Build history of the part. All positions in model axes, mm. A direction names the side the tool comes from. Give positions to 0.01 mm unless a question says otherwise; leave off trailing zeros. Write each loop counter-clockwise with the first axis right and the second up, starting at its lowest first coordinate (ties: lowest second). Pieces come first, ordered by that corner, then holes. Notation, with made-up numbers: M 12.25,2.5 L 62.25,2.5 A20 cw 62.25,35.5 Z; hole C -36,-32 d2. An arc over 180 degrees is marked long. Return JSON: item names as keys, results as strings. Group by question number.
Q1. Band-saw the part on C-C, the plane y = -51.5. Give the cut face in (x, z).
Q2. Pull direction X, two halves, no side cores. Call faces 1 (the flat face through (0, -61.7, -6.5)), 2 (the cylindrical face through (0.315, -61, -16.764)), 3 (the flat face through (-22.5, -57, -19)), 4 (the flat face through (4, -44, -19)): +X half, -X half, draft (parallel to the pull), parting line (faces both ways), or undercut.
Q3. Band-saw the part on B-B, the plane x = -6.5. Give the cut face in (y, z).
Q4. Band-saw the part on D-D, the plane z = -12.5. Give the cut face in (x, y).
Q5. Band-saw the part on A-A, the plane z = -4. Give the cut face in (x, y) (3 decimals), then the cut area to 3 significant figures.
Q6. Tool access for faces 5 (the cylindrical face through (13.9, -62.01, -4.91)), 6 (the flat face through (-14, -63, -4.5)), 7 (the flat face through (0, -45.893, -19)), 8 (the flat face through (14, -63, -4.5)): list every direction of +Z, -Z, +X, -X, +Y, -Y with a clear straight run to the whole face (end or side of a thin tool).
Q7. Flat gauge pins, fed straight in: pin 1 Ø1.9 at (y, z) = (-61, -3.5) entering from -X; pin 2 Ø1.7 at (x, z) = (-2.5, -3.5) entering from +Y; pin 3 Ø1.8 at (x, y) = (-13, -62.5) entering from +Z; pin 4 Ø2.5 at (x, z) = (0, -4) entering from -Y. Where does each tip first touch, or does it go through?
Q8. Wall check: probe 1 along Z at (x, y) = (0, -61.2) (3 decimals); probe 2 along Z at (x, y) = (0, -60.4) (3 decimals); probe 3 along X at (y, z) = (-63.05, -4). Give the ranges that are in metal, low to high.
from build123d import *

# Parameters (mm, degrees)
MODEL_R                   = 8.35
RESSALTO_EXTRUS_O2_DEPTH  = 4
ESBO_O5_W                 = 2
ESBO_O5_H                 = 24
RESSALTO_EXTRUS_O3_DEPTH  = 20
ESBO_O6_OUTSIDE_W         = 30.002
ESBO_O6_OUTSIDE_H         = 34.002
ESBO_O6_OUTSIDE_R         = 13
CORTE_EXTRUS_O1_DEPTH     = 72.292987034
CORTE_EXTRUS_O2_DEPTH     = 72.292987124
RESSALTO_EXTRUS_O4_DEPTH  = 4
CORTE_EXTRUS_O3_DEPTH     = 38.486664414
RESSALTO_EXTRUS_O5_START  = 0.5
RESSALTO_EXTRUS_O5_DEPTH  = 45
RESSALTO_EXTRUS_O6_START  = 0.5
ESBO_O14_R                = 2.115
RESSALTO_EXTRUS_O6_DEPTH  = 3.779219
CORTE_EXTRUS_O4_DEPTH     = 10.1
CORTE_EXTRUS_O7_DEPTH     = 10
ESBO_O17_R                = 3.5
CORTE_EXTRUS_O8_DEPTH     = 2
CORTE_EXTRUS_O11_REACH    = 75.217
ESBO_O19_W                = 67.006666236
ESBO_O19_H                = 28.204946311
CORTE_EXTRUS_O9_DEPTH     = 52.948283002
CORPO_MOVER_COPIAR2_ANGLE = 180


with BuildPart() as part:
    # Model → Ressalto-extrusão2 (new body)
    with BuildSketch(Plane.XY):
        Polygon((0, 44.200000002), (0, 59.200000002), (-5.55, 59.200000002), (-5.55, 63.700000002), (-23, 63.700000002), (-23, 39.700000002), (-5.55, 39.700000002), (-5.55, 44.200000002), align=None)
        with Locations((-13.5, 51.700000002)):
            Circle(MODEL_R, mode=Mode.SUBTRACT)
    extrude(amount=RESSALTO_EXTRUS_O2_DEPTH)

    # Esboço5 → Ressalto-extrusão3 (add)
    with BuildSketch(Plane(origin=(0, 0, 0), x_dir=(-1, 0, 0), z_dir=(0, 0, -1))):
        with Locations((24, 51.700000002)):
            Rectangle(ESBO_O5_W, ESBO_O5_H)
    extrude(amount=-RESSALTO_EXTRUS_O3_DEPTH)

    # Esboço6 outside → Corte-extrusão1 (cut, through all)
    with BuildSketch(Plane.ZY.offset(25)):
        with Locations((10, 51.7)):
            Rectangle(ESBO_O6_OUTSIDE_W, ESBO_O6_OUTSIDE_H)
        with Locations((10, 51.700000002)):
            Circle(ESBO_O6_OUTSIDE_R, mode=Mode.SUBTRACT)
    extrude(amount=-CORTE_EXTRUS_O1_DEPTH, mode=Mode.SUBTRACT)

    # Esboço8 → Corte-extrusão2 (cut, through all)
    with BuildSketch(Plane.ZY.offset(25)):
        Polygon((7.885, 51.700000002), (10, 49.585000002), (12.115, 51.700000002), (10, 53.815000002), align=None)
    extrude(amount=-CORTE_EXTRUS_O2_DEPTH, mode=Mode.SUBTRACT)

    # Espelhar1: part across plane


with BuildPart() as part_1:
    add(part.part)
    add(part.part.mirror(Plane(origin=(0, 44.200000002, 4), x_dir=(0, 0, 1), z_dir=(-1, 0, 0))))

    # Esboço9 → Ressalto-extrusão4 (add)
    with BuildSketch(Plane.XY.offset(4)):
        Polygon((0, 59.200000002), (4, 59.200000002), (4, 44.200000002), (-4, 44.200000002), (-4, 59.200000002), align=None)
    extrude(amount=RESSALTO_EXTRUS_O4_DEPTH)

    # Esboço10 → Corte-extrusão3 (cut, through all)
    with BuildSketch(Plane(origin=(0, 59.200000002, 0), x_dir=(1, 0, 0), z_dir=(0, 1, 0))):
        Polygon((0, -1.885), (-2.115, -4), (0, -6.115), (2.115, -4), align=None)
    extrude(amount=-CORTE_EXTRUS_O3_DEPTH, mode=Mode.SUBTRACT)


with BuildPart() as body_2:
    # Esboço13 → Ressalto-extrusão5 (new body)
    with BuildSketch(Plane.ZY.offset(-23).offset(RESSALTO_EXTRUS_O5_START)):
        with BuildLine():
            Line((18.5, 43.95403331), (18.5, 59.445966694))
            ThreePointArc((18.5, 59.445966694), (16.73742843, 61.019713418), (14.69041576, 62.200000002))
            Line((14.69041576, 62.200000002), (5.30958424, 62.200000002))
            ThreePointArc((5.30958424, 62.200000002), (4.900858659, 62.0077038), (4.5, 61.79950494))
            Line((4.5, 61.79950494), (4.5, 63.479218991))
            ThreePointArc((4.5, 63.479218991), (4.748839551, 63.592237552), (5, 63.700000002))
            Line((5, 63.700000002), (15, 63.700000002))
            ThreePointArc((15, 63.700000002), (17.724005232, 62.156564599), (20, 60.006623865))
            Line((20, 60.006623865), (20, 43.393376139))
            ThreePointArc((20, 43.393376139), (19.281560672, 42.597657914), (18.5, 41.863842216))
            Line((18.5, 41.863842216), (18.5, 43.95403331))
        make_face()
    extrude(amount=RESSALTO_EXTRUS_O5_DEPTH)

    # Esboço14 → Ressalto-extrusão6 (add)
    with BuildSketch(Plane(origin=(0, 59.200000002, 0), x_dir=(1, 0, 0), z_dir=(0, 1, 0)).offset(RESSALTO_EXTRUS_O6_START)):
        Polygon((5.05, -4), (5.05, -8), (5.05, -9.5), (-5.05, -9.5), (-5.05, -8), (-5.05, -4), (-5.05, -0.5), (5.05, -0.5), align=None)
        with Locations(Location((0, -4, 0), (0, 0, 346.325447319))):
            Circle(ESBO_O14_R, mode=Mode.SUBTRACT)
    extrude(amount=RESSALTO_EXTRUS_O6_DEPTH)

    # Esboço15 → Corte-extrusão4 (cut)
    with BuildSketch(Plane(origin=(5.05, 0, 0), x_dir=(0, 0, -1), z_dir=(1, 0, 0))):
        with BuildLine():
            Line((-5.561651151, 63.918881272), (-4.5, 63.918881272))
            Line((-4.5, 63.918881272), (-4.5, 64.979109715))
            Line((-4.5, 64.979109715), (0, 64.979109715))
            Line((0, 64.979109715), (0, 60.006623865))
            ThreePointArc((0, 60.006623865), (-2.520500092, 62.332830346), (-5.561651151, 63.918881272))
        make_face()
    extrude(amount=-CORTE_EXTRUS_O4_DEPTH, mode=Mode.SUBTRACT)

    # Esboço18 → Corte-extrusão7 (cut)
    with BuildSketch(Plane.XY.offset(20)):
        Polygon((-4, 45.893376139), (0, 45.893376139), (4, 45.893376139), (4, 37.813192245), (-4, 37.813192245), align=None)
    extrude(amount=-CORTE_EXTRUS_O7_DEPTH, mode=Mode.SUBTRACT)

    # Esboço17 → Corte-extrusão8 (cut)
    with BuildSketch(Plane(origin=(0, 63.700000002, 0), x_dir=(1, 0, 0), z_dir=(0, 1, 0))):
        with Locations((0, -4)):
            Circle(ESBO_O17_R)
    extrude(amount=-CORTE_EXTRUS_O8_DEPTH, mode=Mode.SUBTRACT)

    # Corte-extrusão11: up to this face of the body (flat: up to its plane)
    corte_extrus_o11_end = Plane(body_2.part.faces().sort_by_distance((-5.05, 61.009194207, 5.162360776))[0])
    # Esboço21 → Corte-extrusão11 (cut, up to the picked face)
    with BuildSketch(Plane(origin=(5.05, 0, 0), x_dir=(0, 0, -1), z_dir=(1, 0, 0)), mode=Mode.PRIVATE) as corte_extrus_o11_sk1:
        with BuildLine():
            Line((-6.115, 59.700000002), (-9.5, 59.700000002))
            Line((-9.5, 59.700000002), (-9.5, 62.200000002))
            ThreePointArc((-9.5, 62.200000002), (-7.531688037, 61.3234494), (-6.115, 59.700000002))
        make_face()
    corte_extrus_o11_tool1 = split(extrude(corte_extrus_o11_sk1.sketch, amount=-CORTE_EXTRUS_O11_REACH, mode=Mode.PRIVATE), bisect_by=corte_extrus_o11_end, keep=Keep.BOTH, mode=Mode.PRIVATE)
    add(corte_extrus_o11_tool1.solids().sort_by(Axis((5.05, 60.667689, 8.211637), (-1, 0, 0)))[0], mode=Mode.SUBTRACT)


with BuildPart() as part_2:
    # Corpo-Mover/Copiar1: moved
    add(part_1.part.moved(Location((0, 0, -38.699148431))))

    # Esboço19 → Corte-extrusão9 (cut, through all)
    with BuildSketch(Plane(origin=(0, 63.700000002, 0), x_dir=(1, 0, 0), z_dir=(0, 1, 0))):
        with Locations((-0.756912401, 28.10560681)):
            Rectangle(ESBO_O19_W, ESBO_O19_H)
    extrude(amount=-CORTE_EXTRUS_O9_DEPTH, mode=Mode.SUBTRACT)


with BuildPart() as body_2_1:
    # Corpo-Mover/Copiar2: moved
    add(body_2.part.rotate(Axis((0, 0, 0), (1, 0, 0)), CORPO_MOVER_COPIAR2_ANGLE))


solid = body_2_1.part
From the geometry:
{
 "1": {"outline": "M -22.5,-20 L 22.5,-20 L 22.5,-18.5 L -22.5,-18.5 Z"},
 "2": {"face 1": "undercut", "face 2": "draft", "face 3": "-X half", "face 4": "undercut"},
 "3": {"outline": "M -63.7,-15 A13 ccw -60.01,-20 L -43.39,-20 A13 ccw -41.86,-18.5 L -59.45,-18.5 A11.5 cw -62.2,-14.69 L -62.2,-5.31 A11.5 cw -61.8,-4.5 L -63.48,-4.5 A13 ccw -63.7,-5 Z"},
 "4": {"outline": "M -22.5,-63.7 L 22.5,-63.7 L 22.5,-62.2 L -22.5,-62.2 Z"},
 "5": {"outline": "M -5.05,-63.233 L -3.5,-63.233 L -3.5,-61.7 L -2.115,-61.7 L -2.115,-59.7 L -5.05,-59.7 Z; M 2.115,-61.7 L 3.5,-61.7 L 3.5,-63.233 L 5.05,-63.233 L 5.05,-59.7 L 2.115,-59.7 Z", "area": "16.5 mm^2"},
 "6": {"face 5": "+X, +Y", "face 6": "+Z, -X, +Y, -Y", "face 7": "+Z, -Z, +Y", "face 8": "+Z, +X, +Y, -Y"},
 "7": {"pin 1": "stops at x = -5.05", "pin 2": "stops at y = -59.7", "pin 3": "stops at z = -4.5", "pin 4": "passes through"},
 "8": {"probe 1": "z = -18.874 to -16.481, -7.371 to -6.115, -1.885 to -1.126", "probe 2": "z = -19.66 to -17.521, -6.578 to -6.115, -1.885 to -0.5", "probe 3": "x = -5.05 to -3.5, 3.5 to 5.05"}
}
